For this review, take the finished solid that the model builds, in its own axes (mm). A direction names the side the tool comes from. Round coordinates to 2 decimals unless told otherwise and drop trailing zeros. Write each loop counter-clockwise with the first axis right and the second up, starting at its lowest first coordinate (ties: lowest second). Pieces come first, ordered by that corner, then holes. Notation, with made-up numbers: (-25, 15.5) - (15, 15.5) arc R27 cw to (15, 54.5) - close; hole circle Ø11 at (-19, -3). An arc over 180 degrees is marked (long way). One line per item, written item: value. Start each with the question number.
Q1. For probe 1 along Y at (x, z) = (37, 7); probe 2 along X at (y, z) = (33, 60.5); probe 3 along Z at (x, y) = (11, 5), list the stretches that pass through material, from the lowest coordinate up.
Q2. Add section C-C on y = 42. Write out the cut boundary in (x, z).
Q3. Mouldability with a two-part tool opening along X and no side actions: class faces 5 (the face through (12.7, 48, -25)), 6 (the face through (0, 25, 45)), 7 (the face through (2, 3, -50.8)) as +X half, -X half, draft (parallel to the pull), parting line (faces both ways), or undercut.
Q4. Tool access review of faces 1 (the face through (6, 44.45, -25)), 2 (the face through (30.23, 49.34, 17.54)), 3 (the face through (46.695, 48, -25)), 4 (the face through (30, 25, 6.35)): name each direction out of +Z, -Z, +X, -X, +Y, -Y from which nothing blocks a thin tool from reaching the whole face with its end or side.
Q5. Add section B-B on x = 27. Write out the cut boundary in (y, z) (3 decimals), and give its area (3 significant figures).
Q6. Add section D-D on z = 51. Write out the cut boundary in (x, y), and give its area (3 significant figures).
Q7. Clearance check with flat-ended pins moving along their axes: pin 1 Ø1 at (x, y) = (39.5, 6) entering from +Z; pin 2 Ø4 at (y, z) = (4, -31) entering from +X; pin 3 Ø6 at (y, z) = (37, 31.5) entering from +X. State where each tip first meets the part, or that it passes through.
Q8. Add section A-A on z = -14. Write out the cut boundary in (x, y), and give its area (3 significant figures).
```python
from build123d import *

# Parameters (mm, degrees)
F0_W         = 50.8
F0_H         = 50.8
F1_DEPTH     = 6.35
F2_W         = 3.2963603735
F2_H         = 5.1404060796
F2_W_2       = 4.6653077006
F2_H_2       = 6.2190000899
F2_W_3       = 4.104912895
F2_H_3       = 6.35
F2_W_4       = 12.7
F3_DEPTH     = 25.4
F4_DEPTH     = 25.4
F5_W         = 10.2360965684
F5_H         = 50.8
F6_DEPTH     = 101.6
F7_W         = 40.5639034316
F7_H         = 4.4053453021
F8_DEPTH     = 12.7
F9_W         = 40.5639034316
F9_H         = 4.8934674442
F10_DEPTH    = 12.7
F11_T1_DEPTH = 53.1514074134
F12_T1_DEPTH = 53.255338931


# Not quite as in the source:
# - a fillet or chamfer that OpenCascade refuses, or shapes differently, is made with other operations: its cross-section is extruded or revolved along the edge and cut away or added


with BuildPart() as f1:
    # F0 (on Top) → F1 (new body)
    with BuildSketch(Plane.XY):
        with Locations((25.4, 25.4)):
            Rectangle(F0_W, F0_H)
    extrude(amount=F1_DEPTH)

    # F2 (on face) → F3 (join)
    with BuildSketch(Plane(origin=(0, 0, 0), x_dir=(1, 0, 0), z_dir=(0, 0, -1))):
        with Locations((48.0348914862, -2.5702030398)):
            Rectangle(F2_W, F2_H)
        with Locations((2.3326538503, -3.109500045)):
            Rectangle(F2_W_2, F2_H_2)
        with Locations((48.7475435525, -47.625)):
            Rectangle(F2_W_3, F2_H_3)
        with Locations((6.35, -47.625)):
            Rectangle(F2_W_4, F2_H_3)
    extrude(amount=F3_DEPTH)

    # F4 (add): faces of the model
    f4_faces = [f1.faces().sort_by_distance(p)[0] for p in [
        (48.0348914862, 2.5702030398, -25.4),
        (2.3326538503, 3.109500045, -25.4),
        (6.35, 47.625, -25.4),
        (48.7475435525, 47.625, -25.4),
    ]]
    extrude(f4_faces, amount=F4_DEPTH)

    # F5 (on face) → F6 (join)
    with BuildSketch(Plane.XY.offset(6.35)):
        with Locations((5.1180482842, 25.4)):
            Rectangle(F5_W, F5_H)
    extrude(amount=F6_DEPTH)

    # F7 (on face) → F8 (join)
    with BuildSketch(Plane.XY.offset(6.35)):
        with Locations((30.5180482842, 2.202672651)):
            Rectangle(F7_W, F7_H)
    extrude(amount=F8_DEPTH)

    # F9 (on face) → F10 (join)
    with BuildSketch(Plane.XY.offset(6.35)):
        with Locations((30.5180482842, 48.3532662779)):
            Rectangle(F9_W, F9_H)
    extrude(amount=F10_DEPTH)

    # F11: fillet of radius 5.08 on 1 edges, made by hand

    # F11_s2 → F11_t1 (cut)
    with BuildSketch(Plane.YZ.offset(10.2360965684)):
        with BuildLine():
            ThreePointArc((4.4053453021, 19.05), (1.2568046175, 17.3600809275), (0, 14.0149984073))
            Line((0, 14.0149984073), (0, 19.05))
            Line((0, 19.05), (4.4053453021, 19.05))
        make_face()
    extrude(amount=F11_T1_DEPTH, mode=Mode.SUBTRACT)

    # F12: fillet of radius 5.08 on 1 edges, made by hand

    # F12_s2 → F12_t1 (cut)
    with BuildSketch(Plane.YZ.offset(10.2360965684)):
        with BuildLine():
            ThreePointArc((45.9065325558, 19.05), (49.3774571346, 17.498962257), (50.8, 13.9734258002))
            Line((50.8, 13.9734258002), (50.8, 19.05))
            Line((50.8, 19.05), (45.9065325558, 19.05))
        make_face()
    extrude(amount=F12_T1_DEPTH, mode=Mode.SUBTRACT)


solid = f1.part
```
Result set:
1. probe 1: y = 0 to 4.41, 45.91 to 50.8
1. probe 2: x = 0 to 10.24
1. probe 3: z = 0 to 6.35
2. outline: (0, 0) - (50.8, 0) - (50.8, 6.35) - (10.24, 6.35) - (10.24, 107.95) - (0, 107.95) - close
3. face 5: undercut
3. face 6: -X half
3. face 7: draft
4. face 1: -Z, +X, -X
4. face 2: +Z, +X, +Y
4. face 3: -Z, +Y
4. face 4: +Z, +X
5. outline: (0, 0) - (50.8, 0) - (50.8, 13.973) arc R5.08 ccw to (45.907, 19.05) - (45.907, 6.35) - (4.405, 6.35) - (4.405, 19.05) arc R5.08 ccw to (0, 14.015) - close
5. area: 430 mm^2
6. outline: (0, 0) - (10.24, 0) - (10.24, 50.8) - (0, 50.8) - close
6. area: 520 mm^2
7. pin 1: stops at z = 6.35
7. pin 2: stops at x = 49.68
7. pin 3: stops at x = 10.24
8. outline: (0, 0) - (4.67, 0) - (4.67, 6.22) - (0, 6.22) - close; (0, 44.45) - (12.7, 44.45) - (12.7, 50.8) - (0, 50.8) - close; (46.39, 0) - (49.68, 0) - (49.68, 5.14) - (46.39, 5.14) - close; (46.7, 44.45) - (50.8, 44.45) - (50.8, 50.8) - (46.7, 50.8) - close
8. area: 153 mm^2
